Work out the finished part from the listing and answer in its coordinate system (mm). Face numbers are marked on the shaded views. A direction names the side the tool comes from. Round coordinates to 2 decimals unless told otherwise and drop trailing zeros. Write each loop counter-clockwise with the first axis right and the second up, starting at its lowest first coordinate (ties: lowest second). Pieces come first, ordered by that corner, then holes.
1. Find section B-B (z = 17). Write down the section's boundary in (x, y), and give its area (3 significant figures).
2. Determine the mould class of the marked faces 1 and 2 for opening direction Y: pulls with the +Y half, pulls with the -Y half, needs draft (parallel to the pull), parting line crosses it, or undercut.
3. Find section C-C (y = 66). Write down the section's boundary in (x, z).
4. Flat-ended cylindrical pins translate along their axes: pin 1 Ø24 at (y, z) = (161, 5) entering from +X; pin 2 Ø3 at (x, z) = (2.5, -8) entering from +Y; pin 3 Ø2 at (x, z) = (2, 14) entering from -Y. Find the tip coordinate at first contact, or state that the pin passes through.
5. Straight lines are drawn through the part: probe 1 along Y at (x, z) = (4.75, -10); probe 2 along X at (y, z) = (33, -20). For each, find the intervals that lie inside material, in ascending order.
6. A tool of negligible diameter and unlimited length cuts with its end or side. For the marked faces 3 and 4, from which of +Z, -Z, +X, -X, +Y, -Y can it reach the whole face along a straight path? Write none if from no direction.
7. Find section A-A (x = 4.5). Write down the section's boundary in (y, z).
```python
from build123d import *

# Parameters (mm, degrees)
SKETCH1_W           = 14
SKETCH1_H           = 90
BOSS_EXTRUDE1_DEPTH = 200
SKETCH2_W           = 10
SKETCH2_H           = 90
CUT_EXTRUDE1_DEPTH  = 206.119477378
SKETCH3_W           = 90
SKETCH3_H           = 1
BOSS_EXTRUDE2_DEPTH = 10


with BuildPart() as part:
    # Sketch1 → Boss-Extrude1 (new body)
    with BuildSketch(Plane(origin=(0, 0, 0), x_dir=(1, 0, 0), z_dir=(0, 1, 0))):
        Rectangle(SKETCH1_W, SKETCH1_H)
    extrude(amount=BOSS_EXTRUDE1_DEPTH)

    # Sketch2 → Cut-Extrude1 (cut, through all)
    with BuildSketch(Plane(origin=(0, 200, 0), x_dir=(1, 0, 0), z_dir=(0, 1, 0))):
        with Locations((2, 0)):
            Rectangle(SKETCH2_W, SKETCH2_H)
    extrude(amount=-CUT_EXTRUDE1_DEPTH, mode=Mode.SUBTRACT)

    # Sketch3 → Boss-Extrude2 (add)
    with BuildSketch(Plane(origin=(-3, 0, 0), x_dir=(0, 0, -1), z_dir=(1, 0, 0))):
        with Locations((0, 120)):
            Rectangle(SKETCH3_W, SKETCH3_H)
        with Locations((0, 80)):
            Rectangle(SKETCH3_W, SKETCH3_H)
    extrude(amount=BOSS_EXTRUDE2_DEPTH)


solid = part.part
```
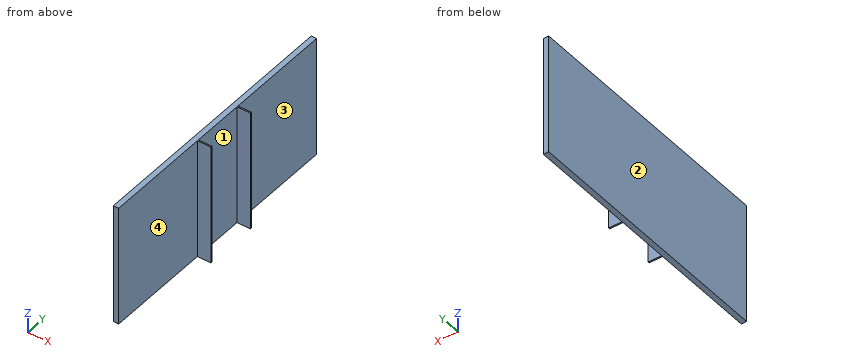
Worked answers:
1. outline: (-7, 0) - (-3, 0) - (-3, 79.5) - (7, 79.5) - (7, 80.5) - (-3, 80.5) - (-3, 119.5) - (7, 119.5) - (7, 120.5) - (-3, 120.5) - (-3, 200) - (-7, 200) - close
1. area: 820 mm2
2. face 1: undercut
2. face 2: needs draft
3. outline: (-7, -45) - (-3, -45) - (-3, 45) - (-7, 45) - close
4. pin 1: stops at x = -3
4. pin 2: stops at y = 120.5
4. pin 3: stops at y = 79.5
5. probe 1: y = 79.5 to 80.5, 119.5 to 120.5
5. probe 2: x = -7 to -3
6. face 3: +Z, -Z, +X, +Y
6. face 4: +Z, -Z, +X, -Y
7. outline: (79.5, -45) - (80.5, -45) - (80.5, 45) - (79.5, 45) - close; (119.5, -45) - (120.5, -45) - (120.5, 45) - (119.5, 45) - close
